Check sheet for the modelled part. Datum: model origin and axes. Units: mm. Face numbers are marked on the shaded views. Give positions to 0.01 mm unless a question says otherwise; leave off trailing zeros. Order: outer loops, then holes, each group sorted by start corner. A loop starts at its lowest first (then second) coordinate and runs counter-clockwise, first axis right, second up.
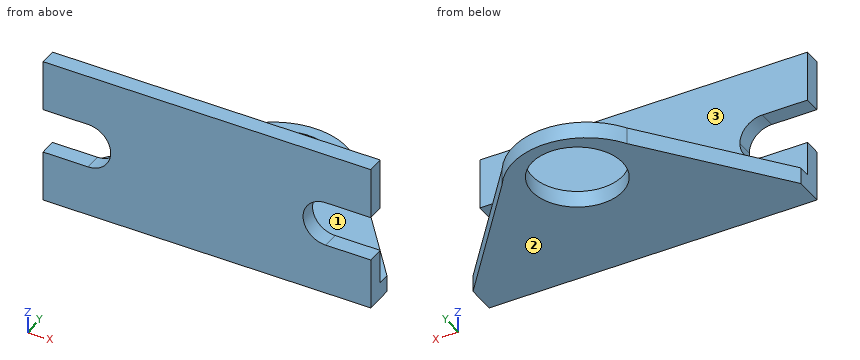
```python
from build123d import *

# Parameters (mm, degrees)
BOSS_EXTRUDE1_DEPTH = 1.778
SKETCH3_R           = 4.826
BOSS_EXTRUDE2_DEPTH = 1.778


with BuildPart() as part:
    # Sketch1 → Boss-Extrude1 (new body)
    with BuildSketch(Plane(origin=(0, 0, 0), x_dir=(1, 0, 0), z_dir=(0, 1, 0))):
        with BuildLine():
            Line((-17.526, 2.413), (-12.7, 2.413))
            ThreePointArc((-12.7, 2.413), (-10.993751337, 1.706248663), (-10.287, 0))
            ThreePointArc((-10.287, 0), (-10.993751337, -1.706248663), (-12.7, -2.413))
            Line((-12.7, -2.413), (-17.526, -2.413))
            Line((-17.526, -2.413), (-17.526, -7.874))
            Line((-17.526, -7.874), (17.526, -7.874))
            Line((17.526, -7.874), (17.526, -2.413))
            Line((17.526, -2.413), (12.7, -2.413))
            ThreePointArc((12.7, -2.413), (10.287, 0), (12.7, 2.413))
            Line((12.7, 2.413), (17.526, 2.413))
            Line((17.526, 2.413), (17.526, 7.874))
            Line((17.526, 7.874), (0, 7.874))
            Line((0, 7.874), (-17.526, 7.874))
            Line((-17.526, 7.874), (-17.526, 2.413))
        make_face()
    extrude(amount=BOSS_EXTRUDE1_DEPTH)

    # Sketch3 → Boss-Extrude2 (add)
    with BuildSketch(Plane(origin=(0, 0, -7.874), x_dir=(-1, 0, 0), z_dir=(0, 0, -1))):
        with BuildLine():
            Line((17.526, 3.048), (6.689775541, 16.597652846))
            ThreePointArc((6.689775541, 16.597652846), (-0.001876966, 20.326885902), (-6.696539897, 16.603059817))
            Line((-6.696539897, 16.603059817), (-17.526, 3.048))
            Line((-17.526, 3.048), (-17.526, 1.778))
            Line((-17.526, 1.778), (17.526, 1.778))
            Line((17.526, 1.778), (17.526, 3.048))
        make_face()
        with Locations((0, 14.224)):
            Circle(SKETCH3_R, mode=Mode.SUBTRACT)
    extrude(amount=-BOSS_EXTRUDE2_DEPTH)


solid = part.part
```
(1) Sectioned sample at D-D (z = 5.25). Enter the section's corners in (x, y), plus the area to 3 significant figures.
(2) Sectioned sample at B-B (z = -6.5). Enter the section's corners in (x, y).
(3) Go/stop test with flat-tipped pins: P1, Ø8, axis at y = 3.5, z = 4, coming from the +X side; P2, Ø1, axis at x = -13, z = 4, coming from the +Y side. Record where each tip stops, or that it passes through.
(4) Sectioned sample at A-A (x = 0). Enter the section's corners in (y, z), plus the area to 3 significant figures.
(5) Thickness scan on L1, parallel to Y at x = 0, z = -7.2; L2, parallel to Y at x = 11.5, z = -4.75; L3, parallel to Z at x = 10, y = 12.25. Record the ranges inside material, lowest first.
(6) Release check for a two-part mould opening along Z. For the marked faces 1, 2 and 3 record: released by +Z, released by -Z, zero draft, split by the parting line, or undercut.
(7) Sectioned sample at C-C (y = 14.75). Enter the section's corners in (x, z), plus the area to 3 significant figures.
Values follow:
1. outline: (-17.53, 0) - (17.53, 0) - (17.53, 1.78) - (-17.53, 1.78) - close
1. area: 62.3 mm2
2. outline: (-17.53, 0) - (17.53, 0) - (17.53, 3.05) - (6.7, 16.6) arc R7.87 ccw to (-6.69, 16.6) - (-17.53, 3.05) - close; hole circle Ø9.65 at (0, 14.22)
3. P1: stops at x = 17.53
3. P2: stops at y = 1.78
4. outline: (0, -7.87) - (9.4, -7.87) - (9.4, -6.1) - (1.78, -6.1) - (1.78, 7.87) - (0, 7.87) - close; (19.05, -7.87) - (20.33, -7.87) - (20.33, -6.1) - (19.05, -6.1) - close
4. area: 43.8 mm2
5. L1: y = 0 to 9.4, 19.05 to 20.33
5. L2: y = 0 to 1.78
5. L3: z = -7.87 to -6.1
6. face 1: released by +Z
6. face 2: released by -Z
6. face 3: zero draft
7. outline: (-8.17, -7.87) - (-4.8, -7.87) - (-4.8, -6.1) - (-8.17, -6.1) - close; (4.8, -7.87) - (8.18, -7.87) - (8.18, -6.1) - (4.8, -6.1) - close
7. area: 12.0 mm2
